from build123d import *

# Parameters (mm, degrees)
SKETCH1_R           = 3
BOSS_EXTRUDE1_DEPTH = 5
FILLET1_R           = 0.4


with BuildPart() as part:
    # Sketch1 → Boss-Extrude1 (new body)
    with BuildSketch(Plane(origin=(0, 0, 0), x_dir=(1, 0, 0), z_dir=(0, 1, 0))):
        Polygon((6.0450921, 0), (3.02254605, 5.235203327), (-3.02254605, 5.235203327), (-6.0450921, 0), (-3.02254605, -5.235203327), (3.02254605, -5.235203327), align=None)
        Circle(SKETCH1_R, mode=Mode.SUBTRACT)
    extrude(amount=BOSS_EXTRUDE1_DEPTH)

    # Sketch2 → Cut-Revolve1 (revolve, cut)
    with BuildSketch(Plane(origin=(0, 0, 0), x_dir=(-0.5, 0, -0.866025404), z_dir=(0.866025404, 0, -0.5))):
        Polygon((-6.389496142, 4.34485452), (-6.038887138, 4.34485452), (-4.919612053, 5), (-6.274952166, 5.0992455), align=None)
    cut_revolve1 = revolve(axis=Axis((0, 0, 0), (0, 1, 0)), mode=Mode.SUBTRACT)

    # Mirror1: Cut-Revolve1 across plane
    add(cut_revolve1.mirror(Plane.ZX.offset(2.5)), mode=Mode.SUBTRACT)

    # Fillet1
    fillet1_edges = [part.edges().sort_by_distance(p)[0] for p in [
        (-3, 0, 0),
        (-3, 5, 0),
    ]]
    fillet(fillet1_edges, radius=FILLET1_R)


solid = part.part
Can you work these out from the model? Positions are in its coordinate system, mm. Give positions to 0.01 mm unless a question says otherwise; leave off trailing zeros. Loops run counter-clockwise (first coordinate to the right, second up) from the corner with the lowest first, then second, coordinate; pieces in that order, holes last. Notation, with made-up numbers: (51.5, 70) - (66.5, 70) arc R25 cw to (66.5, 100) - close; hole circle Ø11 at (84, 79.25). An arc over 180 degrees is marked (long way). Return JSON: item names as keys, results as strings.
1. I'm going to push flat-ended pins straight in: pin 1 Ø1 at (x, z) = (3, 2.5) entering from -Y; pin 2 Ø1 at (y, z) = (3, -1.5) entering from +X; pin 3 Ø1.5 at (y, z) = (2.5, -1) entering from +X. Where does each tip first touch, or does it pass through?
Output values:
{"pin 1": "stops at y = 0", "pin 2": "stops at x = 5.47", "pin 3": "stops at x = 5.9"}
2. If I drill on line 1 (Z direction, x = 0, y = 2.15); line 2 (X direction, y = 0.5, z = 2.5); line 3 (Z direction, x = 2.5, y = 3.5), over which ranges is the centre line in solid material (lowest first)?
Output values:
{"line 1": "z = -5.24 to -3, 3 to 5.24", "line 2": "x = -4.6 to -1.66, 1.66 to 4.6", "line 3": "z = -5.24 to -1.66, 1.66 to 5.24"}
3. We'd pull the mould along X, two halves only. Please class faces 1 (the face through (0, 2, -5.235)), 2 (the face through (-3, 2, 0)), 3 (the face through (4.513, 2.468, 2.654)), 4 (the face through (-4.555, 2.468, 2.581)): +X half, -X half, draft (parallel to the pull), parting line (faces both ways), or undercut.
Output values:
{"face 1": "draft", "face 2": "undercut", "face 3": "+X half", "face 4": "-X half"}
4. I want a section at A-A on x = 0. Please give me the cut outline in (y, z), and give its area (3 significant figures).
Output values:
{"outline": "(0, -4.92) - (0.18, -5.24) - (4.82, -5.24) - (5, -4.92) - (5, -3.4) arc R0.4 ccw to (4.6, -3) - (0.4, -3) arc R0.4 ccw to (0, -3.4) - close; (0, 3.4) arc R0.4 ccw to (0.4, 3) - (4.6, 3) arc R0.4 ccw to (5, 3.4) - (5, 4.92) - (4.82, 5.24) - (0.18, 5.24) - (0, 4.92) - close", "area": "22.1 mm²"}
5. I want a section at B-B on y = 0.8. Please give me the cut outline in (x, z).
Output values:
{"outline": "(-6.05, 0) - (-3.02, -5.24) - (3.02, -5.24) - (6.05, 0) - (3.02, 5.24) - (-3.02, 5.24) - close; hole circle Ø6 at (0, 0)"}
